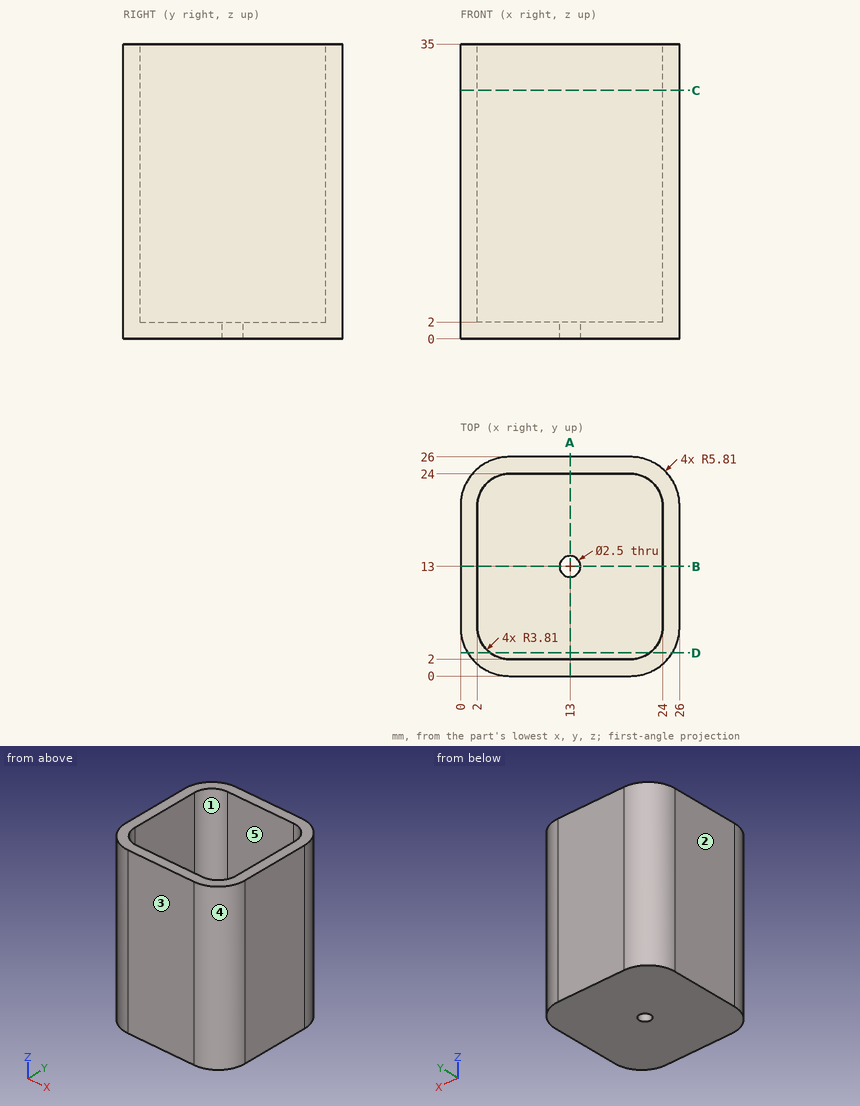
Geometry check sheet. Reference: drawing and pictorial views, mm from the part's lowest x, y, z. A direction names the side the tool comes from. Give positions to 0.01 mm unless a question says otherwise; leave off trailing zeros. Order: outer loops, then holes, each group sorted by start corner. A loop starts at its lowest first (then second) coordinate and runs counter-clockwise, first axis right, second up. Notation, with made-up numbers: (18.25, -19) - (53.25, -19) arc R8 cw to (53.25, -14) - close; hole circle Ø9 at (52.25, 17.25). An arc over 180 degrees is marked (long way). Answer as CSV lines item,"result". Start each with the question number.
Item 1: Section check D-D, the plane y = 2.75. Record the boundary of the cut face in (x, z).
Item 2: Mould release check, pull along X, two halves, no side actions. Record for the marked faces 1, 2 and 3: released by +X, released by -X, zero draft, split by the parting line, or undercut.
Item 3: Section check A-A, the plane x = 13. Record the boundary of the cut face in (y, z).
Item 4: Access from +Z, -Z, +X, -X, +Y, -Y to the whole of each face (thin tool, end or side, straight path). Record for the marked faces 4 and 5.
Item 5: Gauge pin test, flat ends, axial feed: pin 1 (2 mm diameter, centred on x = 14, y = 10.5, fed in from +Z); pin 2 (1.5 mm diameter, centred on x = 2.5, z = 7, fed in from -Y). Record the tip position at first contact, or that the pin passes through.
Item 6: Section check C-C, the plane z = 29.5. Record the boundary of the cut face in (x, y), plus the area to 3 significant figures.
Item 7: Material ranges on L1, parallel to X at y = 13, z = 1.3; L2, parallel to X at y = 11.75, z = 23.5, recorded low to high.
Filled in:
1,outline,"(0.87, 0) - (25.13, 0) - (25.13, 35) - (22.46, 35) - (22.46, 2) - (3.54, 2) - (3.54, 35) - (0.87, 35) - close"
2,face 1,"undercut"
2,face 2,"released by -X"
2,face 3,"zero draft"
3,outline,"(0, 0) - (11.75, 0) - (11.75, 2) - (2, 2) - (2, 35) - (0, 35) - close; (14.25, 0) - (26, 0) - (26, 35) - (24, 35) - (24, 2) - (14.25, 2) - close"
4,face 4,"+Z, -Z, +X, -Y"
4,face 5,"+Z"
5,pin 1,"z = 2"
5,pin 2,"y = 0.59"
6,outline,"(0, 5.81) arc R5.81 ccw to (5.81, 0) - (20.19, 0) arc R5.81 ccw to (26, 5.81) - (26, 20.19) arc R5.81 ccw to (20.19, 26) - (5.81, 26) arc R5.81 ccw to (0, 20.19) - close; hole (2, 5.81) arc R3.81 ccw to (5.81, 2) - (20.19, 2) arc R3.81 ccw to (24, 5.81) - (24, 20.19) arc R3.81 ccw to (20.19, 24) - (5.81, 24) arc R3.81 ccw to (2, 20.19) - close"
6,area,"175 mm^2"
7,L1,"0 to 11.75, 14.25 to 26"
7,L2,"0 to 2, 24 to 26"
